The listing builds one solid part. Answer for the finished solid, in the listing's coordinates (mm). Face numbers are marked on the shaded views. A direction names the side the tool comes from. Give positions to 0.01 mm unless a question says otherwise; leave off trailing zeros. Write each loop counter-clockwise with the first axis right and the second up, starting at its lowest first coordinate (ties: lowest second). Pieces come first, ordered by that corner, then holes.
```python
from build123d import *

# Parameters (mm, degrees)
ESQUISSE3_W                                        = 4
ESQUISSE3_H                                        = 15
CHANFREIN1_SIZE                                    = 0.8
ENL_V_MAT_EXTRU_3_DEPTH                            = 10
CHAMBRAGE_POUR_VIS_T_TE_HEXAGONALE_M31_D           = 3.4
CHAMBRAGE_POUR_VIS_T_TE_HEXAGONALE_M31_DEPTH       = 8
CHAMBRAGE_POUR_VIS_T_TE_HEXAGONALE_M31_CBORE_D     = 5.2
CHAMBRAGE_POUR_VIS_T_TE_HEXAGONALE_M31_CBORE_DEPTH = 3
CHAMBRAGE_POUR_VIS_T_TE_HEXAGONALE_M31_TIP         = 1.021463052
TROU_TARAUD_M31_D                                  = 2.5


with BuildPart() as part:
    # Esquisse1 → Base-R_volution (revolve)
    with BuildSketch(Plane(origin=(0, 0, 0), x_dir=(1, 0, 0), z_dir=(0, 1, 0)), mode=Mode.PRIVATE) as base_r_volution_sk:
        with BuildLine():
            Line((0, 0), (6, 0))
            Line((6, 0), (6, 11.7))
            ThreePointArc((6, 11.7), (5.619238816, 12.619238816), (4.7, 13))
            Line((4.7, 13), (0, 13))
            Line((0, 13), (0, 0))
        make_face()
    revolve(base_r_volution_sk.sketch.rotate(Axis((0, 0, 0), (0, 0, -1)), 180), axis=Axis((0, 0, 0), (0, 0, -1)))

    # Esquisse3 → Boss.-R_vol.1 (revolve)
    with BuildSketch(Plane(origin=(0, 0, 0), x_dir=(1, 0, 0), z_dir=(0, 1, 0))):
        with Locations((2, -7.5)):
            Rectangle(ESQUISSE3_W, ESQUISSE3_H)
    revolve(axis=Axis((0, 0, 0), (0, 0, 1)))

    # Chanfrein1
    chanfrein1_edges = [part.edges().sort_by_distance(p)[0] for p in [
        (-4, 0, 15),
    ]]
    chamfer(chanfrein1_edges, length=CHANFREIN1_SIZE)

    # Esquisse2 → Enl_v. mat.-Extru.3 (cut)
    with BuildSketch(Plane.XY.offset(-13)):
        with BuildLine():
            Line((1.8, -5.723635209), (1.8, 5.723635209))
            ThreePointArc((1.8, 5.723635209), (0, 6), (-1.8, 5.723635209))
            Line((-1.8, 5.723635209), (-1.8, -5.723635209))
            ThreePointArc((-1.8, -5.723635209), (0, -6), (1.8, -5.723635209))
        make_face()
    extrude(amount=ENL_V_MAT_EXTRU_3_DEPTH, mode=Mode.SUBTRACT)

    # Chambrage pour vis _ t_te hexagonale M31
    with Locations(Plane(origin=(7, 0, 0), x_dir=(0, 0, -1), z_dir=(1, 0, 0))):
        with Locations((8, 0)):
            CounterBoreHole(CHAMBRAGE_POUR_VIS_T_TE_HEXAGONALE_M31_D / 2, CHAMBRAGE_POUR_VIS_T_TE_HEXAGONALE_M31_CBORE_D / 2, CHAMBRAGE_POUR_VIS_T_TE_HEXAGONALE_M31_CBORE_DEPTH, depth=CHAMBRAGE_POUR_VIS_T_TE_HEXAGONALE_M31_DEPTH)
            with Locations((0, 0, -(CHAMBRAGE_POUR_VIS_T_TE_HEXAGONALE_M31_DEPTH + CHAMBRAGE_POUR_VIS_T_TE_HEXAGONALE_M31_TIP / 2))):  # 118° drill point
                Cone(0, CHAMBRAGE_POUR_VIS_T_TE_HEXAGONALE_M31_D / 2, CHAMBRAGE_POUR_VIS_T_TE_HEXAGONALE_M31_TIP, mode=Mode.SUBTRACT)

    # Trou taraud_ M31 (through all)
    with Locations(Plane(origin=(-1.8, 0, 0), x_dir=(0, 0, -1), z_dir=(1, 0, 0))):
        with Locations((8, 0)):
            Hole(TROU_TARAUD_M31_D / 2)


solid = part.part
```
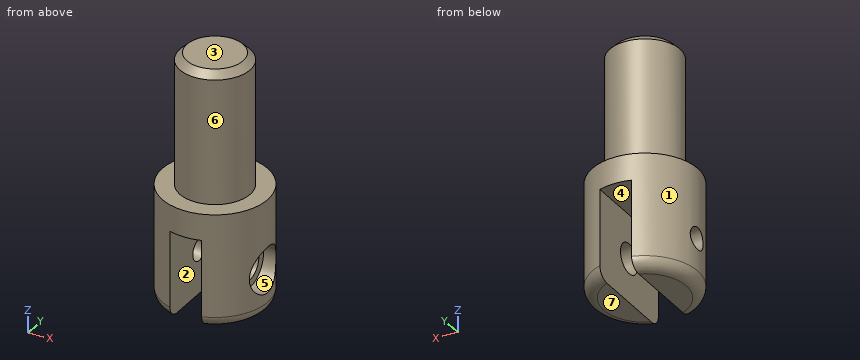
Item 1: A cutting plane is placed at C-C, the plane x = 0. Give the vertices of the cut face in (y, z), plus the area to 3 significant figures.
Conclusion:
outline: (-6, -3) - (6, -3) - (6, 0) - (4, 0) - (4, 14.2) - (3.2, 15) - (-3.2, 15) - (-4, 14.2) - (-4, 0) - (-6, 0) - close
area: 155 mm2
Item 2: Consider probe 1 along Z at (x, y) = (4.5, 0); probe 2 along Z at (x, y) = (-5, 0); probe 3 along Z at (x, y) = (-0.25, -1). Determine where each line is inside the solid, lowest interval first.
Conclusion:
probe 1: z = -13 to -10.6, -5.4 to 0
probe 2: z = -12.96 to -9.25, -6.75 to 0
probe 3: z = -3 to 15
Item 3: A cutting plane is placed at A-A, the plane y = 0. Give the vertices of the cut face in (x, z).
Conclusion:
outline: (-6, -11.7) arc R1.3 ccw to (-4.7, -13) - (-1.8, -13) - (-1.8, -9.25) - (-6, -9.25) - close; (-6, -6.75) - (-1.8, -6.75) - (-1.8, -3) - (1.8, -3) - (1.8, -6.3) - (4, -6.3) - (4, -5.4) - (6, -5.4) - (6, 0) - (4, 0) - (4, 14.2) - (3.2, 15) - (-3.2, 15) - (-4, 14.2) - (-4, 0) - (-6, 0) - close; (1.8, -13) - (4.7, -13) arc R1.3 ccw to (6, -11.7) - (6, -10.6) - (4, -10.6) - (4, -9.7) - (1.8, -9.7) - close
Item 4: A cutting plane is placed at B-B, the plane z = -8. Give the vertices of the cut face in (x, y).
Conclusion:
outline: (-5.87, -1.25) arc R6 ccw to (-1.8, -5.72) - (-1.8, -1.25) - close; (-5.87, 1.25) - (-1.8, 1.25) - (-1.8, 5.72) arc R6 ccw to start; (1.8, -5.72) arc R6 ccw to (5.41, -2.6) - (4, -2.6) - (4, -1.7) - (1.8, -1.7) - close; (1.8, 1.7) - (4, 1.7) - (4, 2.6) - (5.41, 2.6) arc R6 ccw to (1.8, 5.72) - close
Item 5: Which of the six approach directions +Z, -Z, +X, -X, +Y, -Y give full straight-line access (tool end or side, diameter ignored) to the marked faces 4, 5, 6 and 7?
Conclusion:
face 4: -Z, +Y, -Y
face 5: +X
face 6: +Z
face 7: -Z, +X, -X, +Y, -Y
Item 6: Determine the mould class of the marked faces 1, 2 and 3 for opening direction X: pulls with the +X half, pulls with the -X half, needs draft (parallel to the pull), parting line crosses it, or undercut.
Conclusion:
face 1: parting line crosses it
face 2: undercut
face 3: needs draft
Item 7: A cutting plane is placed at D-D, the plane z = 3.75. Give the vertices of the cut face in (x, y), plus the area to 3 significant figures.
Conclusion:
outline: circle Ø8 at (0, 0)
area: 50.3 mm2
Item 8: Each of these flat-tipped pins is pushed along its axis until it touches: P1, Ø4.5, axis at y = 0, z = -8, coming from the +X side; P2, Ø1, axis at x = 1, z = 6.5, coming from the -Y side; P3, Ø5, axis at y = 2.5, z = -8, coming from the +X side. Where does it stop, or does it pass through?
Conclusion:
P1: stops at x = 4
P2: stops at y = -3.97
P3: stops at x = 5.85
